Check sheet for the modelled part. Datum: model origin and axes. Units: mm. A direction names the side the tool comes from. Give positions to 0.01 mm unless a question says otherwise; leave off trailing zeros. Loops run counter-clockwise (first coordinate to the right, second up) from the corner with the lowest first, then second, coordinate; pieces in that order, holes last. Notation, with made-up numbers: (32.5, 74) - (62.5, 74) arc R12 cw to (62.5, 84) - close; hole circle Ø10 at (-22.5, 65.5). An arc over 180 degrees is marked (long way). Answer in a Markdown table with one row per item. Add a question column.
(1) Thickness scan on L1, parallel to X at y = 6.5, z = 27; L2, parallel to Z at x = 56, y = 14.5; L3, parallel to Z at x = 23.5, y = 6. Record the ranges inside material, lowest first.
(2) Sectioned sample at A-A on y = 9. Enter the section's corners in (x, z), then the cut area to 3 significant figures.
(3) Sectioned sample at B-B on z = 49.5. Enter the section's corners in (x, y), then the cut area to 3 significant figures.
(4) Go/stop test with flat-tipped pins: P1, Ø7, axis at x = 42.5, y = 34.5, coming from the +Z side; P2, Ø3, axis at x = 7, z = 40.5, coming from the -Y side; P3, Ø2, axis at x = 69.5, z = 42.5, coming from the -Y side. Record where each tip stops, or that it passes through.
(5) Draft check along X on faces 1 (the face through (0, 29, 32)), 2 (the face through (60.008, 19, 64)), 3 (the face through (51.34, 41.527, 32.349)), 4 (the face through (34, 23, 0)). Enter one of: released by +X, released by -X, zero draft, split by the parting line, or undercut.
(6) Sectioned sample at D-D on z = 18.5. Enter the section's corners in (x, y).
(7) Set-up check for faces 5 (the face through (33.795, 40.928, 21.746)), 6 (the face through (44, 18, 55.166)), 7 (the face through (44, 0, 57)), 8 (the face through (44, 20, 59.267)), 9 (the face through (14, 29, 65.617)): record each of +Z, -Z, +X, -X, +Y, -Y from which the full face is reachable in a straight line by a thin tool's end or side.
(8) Sectioned sample at C-C on x = 53.5. Enter the section's corners in (y, z), then the cut area to 3 significant figures.
Autodesk Inventor part; units mm, degrees
ref_plane "YZ Plane" through (0, 0, 0) normal (1, 0, 0) x (0, 1, 0)
ref_plane "XZ Plane" through (0, 0, 0) normal (0, 1, 0) x (-1, 0, 0)
ref_plane "XY Plane" through (0, 0, 0) normal (0, 0, 1) x (1, 0, 0)
sketch "Sketch1" plane through (0, 0, 0) normal (0, 0, 1) x (1, 0, 0)
  line L0 (0, 0) -> (0, 59.2667)
  line L1 (0, 59.2667) -> (14.8167, 59.2667)
  line L2 (14.8167, 59.2667) -> (88.9, 23.2833)
  line L3 (88.9, 23.2833) -> (88.9, 0)
  line L4 (88.9, 0) -> (0, 0)
  dimension "OverallHeight" = 59.2667
  dimension "TopWidth" = 14.8167
  dimension "RightHeight" = 23.2833
  dimension "OverallWidth" = 88.9
extrude "Extrusion1" add sketch "Sketch1" along normal blind 65.6167
sketch "Sketch2" plane through (14.8167, 59.2667, 65.6167) normal (0.436904, 0.8995082, 0) x (0.8995082, -0.436904, 0)
  circle A0 centre (25.2098, 43.7444) radius 8.9958
  circle A1 centre (66.4848, 43.7444) radius 8.2021
  line L0 (0, 65.6167) -> (82.3598, 65.6167)
  line L1 (82.3598, 65.6167) -> (82.3598, 0)
  point P0 (12.5661, 65.6167)
  dimension "UpperHoleDiameter" = 17.9917
  dimension "LowerHoleDiameter" = 16.4042
  dimension "EdgeDistance" = 15.875
  dimension "HoleAllignment" = 0
  dimension "HoleToCenter" = 41.275
  dimension "BackEdgeToHoleCenters" = 21.8722
extrude "Extrusion2" cut sketch "Sketch2" against normal blind 8.2021
sketch "Sketch3" plane through (14.8167, 59.2667, 65.6167) normal (0.436904, 0.8995082, 0) x (0.8995082, -0.436904, 0)
  line L0 (82.3598, 0) -> (0, 0)
  line L1 (22.3523, 0) -> (53.4673, 0)
  line L2 (26.0565, 6.35) -> (49.7632, 6.35)
  line L3 (22.3523, 0) -> (22.3523, 2.6458)
  line L4 (53.4673, 2.6458) -> (53.4673, 0)
  line L5 (82.3598, 65.6167) -> (82.3598, 0)
  arc A0 (26.0565, 6.35) -> (22.3523, 2.6458) centre (26.0565, 2.6458) ccw
  arc A1 (53.4673, 2.6458) -> (49.7632, 6.35) centre (49.7632, 2.6458) ccw
  point P0 (12.5661, 65.6167)
  dimension "NotchWidth" = 31.115
  dimension "NotchDepth" = 6.35
  dimension "NotchLocation" = 28.8925
  dimension "d18" = 3.7042
sketch "Sketch4" plane through (0, 59.2667, 0) normal (0, 1, 0) x (1, 0, 0)
  line L0 (88.9, -65.6167) -> (0, -65.6167)
  line L1 (28.8925, -65.6167) -> (60.0075, -65.6167)
  line L2 (32.5967, -59.2667) -> (56.3033, -59.2667)
  line L3 (28.8925, -65.6167) -> (28.8925, -62.9708)
  line L4 (60.0075, -62.9708) -> (60.0075, -65.6167)
  line L5 (88.9, 57.15) -> (88.9, -65.6167)
  arc A0 (32.5967, -59.2667) -> (28.8925, -62.9708) centre (32.5967, -62.9708) ccw
  arc A1 (60.0075, -62.9708) -> (56.3033, -59.2667) centre (56.3033, -62.9708) ccw
  line L6 (14.8167, -65.6167) -> (0, -65.6167)
  line L7 (88.9, 0) -> (88.9, -65.6167)
  point P0 (0, 0)
  point P1 (11.3592, 57.15)
  dimension "d19" = 31.115
  dimension "d20" = 6.35
  dimension "d21" = 28.8925
  dimension "d22" = 3.7042
  dimension "d26" = 0
  dimension "d27" = 0
extrude "Extrusion3" cut sketch "Sketch4" against normal through all
shell "Shell1" thickness 4.101 removed faces 1 at (40.4989, 0, 19.7556)
equation "\"OverallWidth\" = 1.5 * OverallHeight"
equation "\"BackEdgeToHoleCenters\" = 0.333333 * Depth"
equation "\"HoleDepth\" = 0.5 * LowerHoleDiameter"
equation "\"NotchWidth\" = 0.35 * OverallWidth"
equation "\"NotchLocation\" = 0.5 * OverallWidth - 0.5 * NotchWidth"
equation "\"d18\" = 0.25 * TopWidth"
equation "\"d19\" = 0.35 * OverallWidth"
equation "\"d21\" = 0.5 * OverallWidth - 0.5 * d19"
equation "\"d22\" = 0.25 * TopWidth"
equation "\"d28\" = 0.5 * LowerHoleDiameter"
equation "\"ShellThickness\" = 0.5 * HoleDepth"
equation "\"d23\" = 1.5 * OverallHeight"
equation "\"d24\" = TopWidth"
equation "\"d25\" = OverallHeight"
properties part number "8.2 Q2" material "Aluminum 6061"
Reply:
| question | item | result |
|---|---|---|
| 1 | L1 | 0 to 4.1, 84.8 to 88.9 |
| 1 | L2 | 0 to 4.1, 55.17 to 59.27 |
| 1 | L3 | 0 to 4.1, 61.52 to 65.62 |
| 2 | outline | (0, 0) - (88.9, 0) - (88.9, 65.62) - (60.01, 65.62) - (60.01, 62.97) arc R3.7 cw to (56.3, 59.27) - (32.6, 59.27) arc R3.7 cw to (28.89, 62.97) - (28.89, 65.62) - (0, 65.62) - close; hole (4.1, 4.1) - (84.8, 4.1) - (84.8, 61.52) - (63.97, 61.52) arc R7.81 cw to (56.3, 55.17) - (32.6, 55.17) arc R7.81 cw to (24.93, 61.52) - (4.1, 61.52) - close |
| 2 | area | 1,230 mm^2 |
| 3 | outline | (0, 0) - (4.1, 0) - (4.1, 55.17) - (13.87, 55.17) - (84.8, 20.72) - (84.8, 0) - (88.9, 0) - (88.9, 23.28) - (14.82, 59.27) - (0, 59.27) - close |
| 3 | area | 706 mm^2 |
| 4 | P1 | z = 59.27 |
| 4 | P2 | y = 55.17 |
| 4 | P3 | y = 27.66 |
| 5 | face 1 | released by -X |
| 5 | face 2 | undercut |
| 5 | face 3 | released by +X |
| 5 | face 4 | zero draft |
| 6 | outline | (0, 0) - (4.1, 0) - (4.1, 55.17) - (13.87, 55.17) - (24.32, 50.09) - (20.73, 42.71) - (43.5, 31.65) - (47.08, 39.03) - (62.19, 31.7) - (58.6, 24.32) - (79.89, 13.98) - (83.47, 21.36) - (84.8, 20.72) - (84.8, 0) - (88.9, 0) - (88.9, 23.28) - (81.35, 26.95) - (77.76, 19.57) - (64.31, 26.11) - (67.89, 33.49) - (44.99, 44.61) - (41.41, 37.23) - (26.41, 44.52) - (29.99, 51.9) - (14.82, 59.27) - (0, 59.27) - close |
| 7 | face 5 | none |
| 7 | face 6 | -Y |
| 7 | face 7 | +Z, -Z, +X, -X, -Y |
| 7 | face 8 | +Z, +Y, -Y |
| 7 | face 9 | +Z, +X, -X, +Y, -Y |
| 8 | outline | (0, 0) - (40.48, 0) - (40.48, 59.27) - (0, 59.27) - (0, 55.17) - (35.92, 55.17) - (35.92, 4.1) - (0, 4.1) - close |
| 8 | area | 565 mm^2 |
